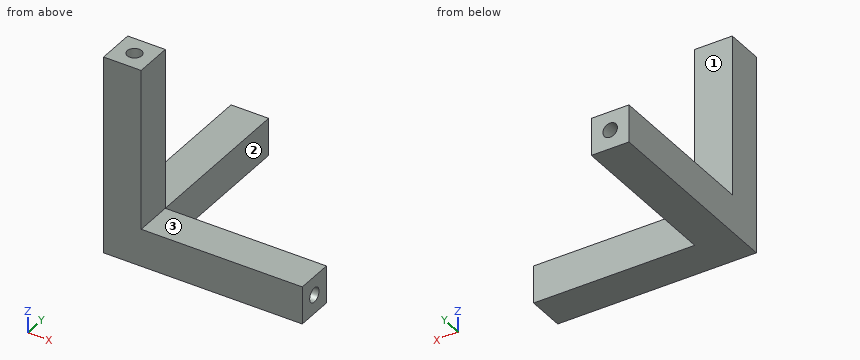
from build123d import *

# Parameters (mm, degrees)
BOSS_EXTRUDE1_DEPTH  = 1.75
SKETCH3_R            = 0.675
CUT_EXTRUDE1_DEPTH   = 15
SKETCH4_R            = 0.675
CUT_EXTRUDE2_DEPTH   = 15
SKETCH5_W            = 3.5
SKETCH5_H            = 3.5
CUT_SWEEP1_PROFILE_R = 0.675


with BuildPart() as part:
    # Sketch2 → Boss-Extrude1 (new body, symmetric)
    with BuildSketch(Plane(origin=(0, 0, 0), x_dir=(1, 0, 0), z_dir=(0, 1, 0))):
        Polygon((-1.75, 1.75), (-1.75, -16.75), (1.75, -16.75), (1.75, -1.75), (16.75, -1.75), (16.75, 1.75), align=None)
    extrude(amount=BOSS_EXTRUDE1_DEPTH, both=True)

    # Sketch3 → Cut-Extrude1 (cut)
    with BuildSketch(Plane.XY.offset(16.75)):
        Circle(SKETCH3_R)
    extrude(amount=-CUT_EXTRUDE1_DEPTH, mode=Mode.SUBTRACT)

    # Sketch4 → Cut-Extrude2 (cut)
    with BuildSketch(Plane(origin=(16.75, 0, 0), x_dir=(0, 0, -1), z_dir=(1, 0, 0))):
        Circle(SKETCH4_R)
    extrude(amount=-CUT_EXTRUDE2_DEPTH, mode=Mode.SUBTRACT)

    # Sweep1: sweep along a path in Sketch7
    with BuildLine(Plane(origin=(0, 0, 0), x_dir=(0.707106781, 0, 0.707106781), z_dir=(-0.707106781, 0, 0.707106781))) as sweep1_path:
        Line((0, 1.75), (0, 16.75))
    # Sketch5 → Sweep1 (sweep)
    with BuildSketch(Plane(origin=(0, 1.75, 0), x_dir=(1, 0, 0), z_dir=(0, 1, 0))):
        Rectangle(SKETCH5_W, SKETCH5_H)
    sweep(path=sweep1_path.line)

    # Cut-Sweep1: sweep along a path in Sketch7_2
    with BuildLine(Plane(origin=(0, 0, 0), x_dir=(0.707106781, 0, 0.707106781), z_dir=(-0.707106781, 0, 0.707106781))) as cut_sweep1_path:
        Line((0, 1.75), (0, 16.75))
    # Cut-Sweep1 profile (on start of the path) → Cut-Sweep1 (sweep, cut)
    with BuildSketch(Plane(origin=(0, 1.75, 0), x_dir=(1, 0, 0), z_dir=(0, 1, 0))):
        Circle(CUT_SWEEP1_PROFILE_R)
    sweep(path=cut_sweep1_path.line, mode=Mode.SUBTRACT)


solid = part.part
Could you check a few things on this model? Use its own coordinates, in mm. Face numbers are marked on the shaded views. A direction names the side the tool comes from. Give positions to 0.01 mm unless a question says otherwise; leave off trailing zeros. Loops run counter-clockwise (first coordinate to the right, second up) from the corner with the lowest first, then second, coordinate; pieces in that order, holes last. Notation, with made-up numbers: (87, 31) -> (139, 31) arc R18 cw to (139, 48) -> close; hole circle Ø7 at (67.5, 53.5). An arc over 180 degrees is marked (long way). Answer as CSV lines item,"result". Start each with the question number.
(1) If we section it at B-B on x = 10.5: Write out the boundary of the cut face in (y, z) (3 decimals).
(2) I need wall thicknesses on probe 1 along Y at (x, z) = (9, 0) (3 decimals); probe 2 along Y at (x, z) = (-0.25, 9.5). Which ranges of each line are inside material? Lowest first, please.
(3) Which directions (+Z, -Z, +X, -X, +Y, -Y) give clear straight access to the entire face, cutting with the end or side of a thin tool? Please do the marked faces 1, 2 and 3.
(4) If we section it at A-A on y = 0: Write out the boundary of the cut face in (x, z) (3 decimals).
(5) I'm going to push flat-ended pins straight in: pin 1 Ø3 at (y, z) = (6.5, 0.5) entering from +X; pin 2 Ø4 at (x, y) = (9, 0) entering from +Z; pin 3 Ø8 at (x, y) = (6, 6.5) entering from +Z; pin 4 Ø3 at (x, z) = (0, 12) entering from +Y. Where does each tip first touch, or does it pass through?
Computed:
1,outline,"(-1.75, -1.75) -> (1.75, -1.75) -> (1.75, 1.75) -> (-1.75, 1.75) -> close; hole circle Ø1.35 at (0, 0)"
2,probe 1,"y = -1.75 to -0.675, 0.675 to 1.75"
2,probe 2,"y = -1.75 to -0.63, 0.63 to 1.75"
3,face 1,"+Z, +X, -X, +Y"
3,face 2,"+Z, -Z, +X, +Y"
3,face 3,"+Z, +X, +Y, -Y"
4,outline,"(-1.75, -1.75) -> (16.75, -1.75) -> (16.75, -0.675) -> (1.75, -0.675) -> (1.75, 0.675) -> (16.75, 0.675) -> (16.75, 1.75) -> (1.75, 1.75) -> (1.75, 16.75) -> (0.675, 16.75) -> (0.675, 1.75) -> (-0.675, 1.75) -> (-0.675, 16.75) -> (-1.75, 16.75) -> close"
5,pin 1,"stops at x = 1.75"
5,pin 2,"stops at z = 1.75"
5,pin 3,"passes through"
5,pin 4,"stops at y = 1.75"
